from build123d import *

# Parameters (mm, degrees)
F0_R     = 5
F2_DEPTH = 9
F1_R     = 4.5
F3_DEPTH = 19
F6_R     = 3
F7_DEPTH = 38


with BuildPart() as f2:
    # F0 (on Front) → F2 (new body)
    with BuildSketch(Plane.XZ):
        Circle(F0_R)
    extrude(amount=F2_DEPTH)

    # F1 (on face) → F3 (join)
    with BuildSketch(Plane.XZ):
        Circle(F1_R)
    extrude(amount=F3_DEPTH)

    # F5: F2 across plane


with BuildPart() as f2_1:
    add(f2.part)
    add(f2.part.mirror(Plane.XZ.offset(19)))

    # F6 (on face) → F7 (cut)
    with BuildSketch(Plane(origin=(0, 0, 0), x_dir=(-1, 0, 0), z_dir=(0, 1, 0))):
        Circle(F6_R)
    extrude(amount=-F7_DEPTH, mode=Mode.SUBTRACT)


solid = f2_1.part
Source: CAD feature listing. Evaluate the final solid. Frame: model axes, mm. Round coordinates to 2 decimals unless told otherwise and drop trailing zeros. Order: outer loops, then holes, each group sorted by start corner. A loop starts at its lowest first (then second) coordinate and runs counter-clockwise, first axis right, second up. Notation, with made-up numbers: (47.5, -21.75) -> (75.5, -21.75) arc R30 ccw to (75.5, 2.25) -> close; hole circle Ø5 at (79.25, -13.5). An arc over 180 degrees is marked (long way). Answer as CSV lines item,"result".
Item 1: Pin query (flat end, axial travel): pin 1 Ø5 at (x, y) = (-1, -22.5) entering from -Z; pin 2 Ø1.5 at (x, y) = (-2.5, -26) entering from -Z; pin 3 Ø3 at (y, z) = (-9.5, 2.5) entering from -X. Return the tip coordinate at first contact, or that it passes through.
A:
pin 1,"z = -4.5"
pin 2,"z = -4.15"
pin 3,"x = -4.88"
Item 2: Pull-direction query (Y, two-part tool) for faces 1 (the face through (-0.59, -19.14, 4.46)), 2 (the face through (-0.1, 0, -3.3)), 3 (the face through (-1.08, -33.56, -4.88)); classes: pulls with the +Y half, pulls with the -Y half, needs draft (parallel to the pull), parting line crosses it, or undercut.
A:
face 1,"undercut"
face 2,"pulls with the +Y half"
face 3,"needs draft"
Item 3: Section B-B, the plane z = 0. Return loops of the section in (x, y), plus the area to 3 significant figures.
A:
outline,"(-5, -38) -> (-3, -38) -> (-3, 0) -> (-5, 0) -> (-5, -9) -> (-4.5, -9) -> (-4.5, -29) -> (-5, -29) -> close; (3, -38) -> (5, -38) -> (5, -29) -> (4.5, -29) -> (4.5, -9) -> (5, -9) -> (5, 0) -> (3, 0) -> close"
area,"132 mm²"
Item 4: Line query: L1, parallel to Z at x = 0, y = -23.5; L2, parallel to Y at x = -3.75, z = -2.75; L3, parallel to Z at x = 0, y = -8.5. Output: solid intervals per line, ascending.
A:
L1,"-4.5 to -3, 3 to 4.5"
L2,"-38 to -29, -9 to 0"
L3,"-5 to -3, 3 to 5"
Item 5: Section A-A, the plane x = 0. Return loops of the section in (y, z).
A:
outline,"(-38, -5) -> (-29, -5) -> (-29, -4.5) -> (-9, -4.5) -> (-9, -5) -> (0, -5) -> (0, -3) -> (-38, -3) -> close; (-38, 3) -> (0, 3) -> (0, 5) -> (-9, 5) -> (-9, 4.5) -> (-29, 4.5) -> (-29, 5) -> (-38, 5) -> close"
Item 6: Section D-D, the plane x = 3.75. Return loops of the section in (y, z), plus the area to 3 significant figures.
A:
outline,"(-38, -3.31) -> (-29, -3.31) -> (-29, -2.49) -> (-9, -2.49) -> (-9, -3.31) -> (0, -3.31) -> (0, 3.31) -> (-9, 3.31) -> (-9, 2.49) -> (-29, 2.49) -> (-29, 3.31) -> (-38, 3.31) -> close"
area,"219 mm²"
Item 7: Section C-C, the plane y = -12. Return loops of the section in (x, z), plus the area to 3 significant figures.
A:
outline,"circle Ø9 at (0, 0); hole circle Ø6 at (0, 0)"
area,"35.3 mm²"
